```python
from build123d import *

# Parameters (mm, degrees)
BOSS_EXTRUDE1_DEPTH = 26
SKETCH2_R           = 5
SKETCH2_R_2         = 1.75
CUT_EXTRUDE1_DEPTH  = 26
FILLET1_R           = 13
SKETCH4_R           = 4
SKETCH4_R_2         = 1.6
CUT_EXTRUDE2_DEPTH  = 26
FILLET2_R           = 1
FILLET3_R           = 4
FILLET4_R           = 2
CHAMFER1_SIZE       = 1


with BuildPart() as part:
    # Sketch1 → Boss-Extrude1 (new body)
    with BuildSketch(Plane(origin=(0, 0, 0), x_dir=(1, 0, 0), z_dir=(0, 1, 0))):
        Polygon((0, 0), (0, 33), (-3, 33), (-3, 3), (-33, 3), (-33, 0), align=None)
    extrude(amount=BOSS_EXTRUDE1_DEPTH)

    # Sketch2 → Cut-Extrude1 (cut)
    with BuildSketch(Plane.XY):
        with Locations((-16.5, 13)):
            Circle(SKETCH2_R)
        with Locations((-24.5, 21)):
            Circle(SKETCH2_R_2)
        with Locations((-8.5, 21)):
            Circle(SKETCH2_R_2)
        with Locations((-8.5, 5)):
            Circle(SKETCH2_R_2)
        with Locations((-24.5, 5)):
            Circle(SKETCH2_R_2)
    extrude(amount=-CUT_EXTRUDE1_DEPTH, mode=Mode.SUBTRACT)

    # Fillet1
    fillet1_edges = [part.edges().sort_by_distance(p)[0] for p in [
        (-1.5, 0, -33),
        (-1.5, 26, -33),
    ]]
    fillet(fillet1_edges, radius=FILLET1_R - 0.0001)  # a hair under: the kernel refuses the full size

    # Sketch4 → Cut-Extrude2 (cut)
    with BuildSketch(Plane(origin=(0, 0, 0), x_dir=(0, 0, -1), z_dir=(1, 0, 0))):
        with Locations((20, 13)):
            Circle(SKETCH4_R)
        with Locations((20, 21.5)):
            Circle(SKETCH4_R_2)
        with Locations((20, 4.5)):
            Circle(SKETCH4_R_2)
    extrude(amount=-CUT_EXTRUDE2_DEPTH, mode=Mode.SUBTRACT)

    # Fillet2
    fillet2_edges = [part.edges().sort_by_distance(p)[0] for p in [
        (-3, 13, -3),
    ]]
    fillet(fillet2_edges, radius=FILLET2_R)

    # Fillet3
    fillet3_edges = [part.edges().sort_by_distance(p)[0] for p in [
        (0, 13, 0),
    ]]
    fillet(fillet3_edges, radius=FILLET3_R)

    # Fillet4
    fillet4_edges = [part.edges().sort_by_distance(p)[0] for p in [
        (-33, 26, -1.5),
        (-33, 0, -1.5),
    ]]
    fillet(fillet4_edges, radius=FILLET4_R)

    # Chamfer1
    chamfer1_edges = [part.edges().sort_by_distance(p)[0] for p in [
        (0, 4.5, -18.4),
        (0, 21.5, -18.4),
    ]]
    chamfer(chamfer1_edges, length=CHAMFER1_SIZE)


solid = part.part
```
Build history of the part. All positions in model axes, mm. A direction names the side the tool comes from. Coordinates: 2 decimals unless noted, no trailing zeros. Order: outer loops, then holes, each group sorted by start corner. A loop starts at its lowest first (then second) coordinate and runs counter-clockwise, first axis right, second up. Notation, with made-up numbers: M 82,-32.75 L 118,-32.75 A17 cw 118,-8.75 Z; hole C -5.75,-2 d7. An arc over 180 degrees is marked long. One line per question, with ' | ' between items. Start each with the question number.
1. Wall check: line 1 along Y through (x, z) = (-8.5, -1.15); line 2 along Y through (x, z) = (-1, -20); line 3 along Z through (x, y) = (-19, 21.75). Give the ranges that are in metal, low to high. Write a range as [from, to].
2. Cut at B-B (x = -16.5). Write the cut outline in (y, z), plus the area to 3 significant figures.
3. Flat gauge pins, fed straight in: P1, Ø7, axis at y = 13, z = -20, coming from the -X side; P2, Ø13, axis at x = -22, y = 9, coming from the -Z side; P3, Ø3.5, axis at y = 21.5, z = -20, coming from the -X side. Where does each tip first touch, or does it go through?
4. Mould opens along Y. For faces 3 (the face through (-3.285, 13.182, -3.301)), 4 (the face through (-25.89, 3.94, -1.48)), 5 (the face through (-32.43, 25.4, -1.48)) say: +Y half, -Y half, draft (parallel to the pull), parting line (faces both ways), or undercut.
5. Cut at C-C (y = 4.5). Write the cut outline in (x, z).
6. Cut at A-A (x = -8.5). Write the cut outline in (y, z).
7. Tool access for faces 1 (the face through (-22, 13, -3)), 2 (the face through (-25.79, 22.18, -1.48)): list every direction of +Z, -Z, +X, -X, +Y, -Y with a clear straight run to the whole face (end or side of a thin tool).
8. Cut at D-D (y = 11.75). Write the cut outline in (x, z).
The answers:
1) line 1: y = [0, 3.25], [6.75, 19.25], [22.75, 26] | line 2: y = [0, 2.9], [6.1, 9], [17, 19.9], [23.1, 26] | line 3: z = [-3, 0]
2) outline: M 0,-3 L 8,-3 L 8,0 L 0,0 Z; M 18,-3 L 26,-3 L 26,0 L 18,0 Z | area: 48.0 mm2
3) P1: passes through | P2: stops at z = -3 | P3: stops at x = -3
4) face 3: draft | face 4: undercut | face 5: +Y half
5) outline: M -33,-3 L -26.18,-3 L -26.18,0 L -33,0 Z; M -22.82,-3 L -10.18,-3 L -10.18,0 L -22.82,0 Z; M -6.82,-3 L -4,-3 A1 cw -3,-4 L -3,-18.4 L -1,-18.4 L 0,-17.4 L 0,-4 A4 ccw -4,0 L -6.82,0 Z; M -3,-29.84 L 0,-29.84 L 0,-22.6 L -1,-21.6 L -3,-21.6 Z
6) outline: M 0,-3 L 3.25,-3 L 3.25,0 L 0,0 Z; M 6.75,-3 L 19.25,-3 L 19.25,0 L 6.75,0 Z; M 22.75,-3 L 26,-3 L 26,0 L 22.75,0 Z
7) face 1: -Z, -X, +Y, -Y | face 2: +Z, -Z
8) outline: M -33,-3 L -21.34,-3 L -21.34,0 L -33,0 Z; M -11.66,-3 L -4,-3 A1 cw -3,-4 L -3,-16.2 L 0,-16.2 L 0,-4 A4 ccw -4,0 L -11.66,0 Z; M -3,-32.94 L 0,-32.94 L 0,-23.8 L -3,-23.8 Z
